```python
from build123d import *

# Parameters (mm, degrees)
CROQUIS1_R              = 3
SALIENTE_EXTRUIR1_DEPTH = 30
CROQUIS2_W              = 3.201408756
CROQUIS2_H              = 4
SALIENTE_EXTRUIR2_DEPTH = 9
REDONDEO2_R             = 1.5


with BuildPart() as part:
    # Croquis1 → Saliente-Extruir1 (new body)
    with BuildSketch(Plane(origin=(0, 0, 0), x_dir=(1, 0, 0), z_dir=(0, 1, 0))):
        with Locations(Location((0, 0, 0), (0, 0, 270))):
            Circle(CROQUIS1_R)
    extrude(amount=SALIENTE_EXTRUIR1_DEPTH)

    # Croquis2 → Saliente-Extruir2 (add)
    with BuildSketch(Plane.XY):
        with Locations((0, 28)):
            Rectangle(CROQUIS2_W, CROQUIS2_H)
    extrude(amount=SALIENTE_EXTRUIR2_DEPTH)

    # Redondeo2
    redondeo2_edges = [part.edges().sort_by_distance(p)[0] for p in [
        (1.600704378, 28, 9),
        (-1.600704378, 28, 9),
    ]]
    fillet(redondeo2_edges, radius=REDONDEO2_R)


solid = part.part
```
Geometry check sheet. Reference: the model listing, model coordinates, mm. A direction names the side the tool comes from. Give positions to 0.01 mm unless a question says otherwise; leave off trailing zeros. Order: outer loops, then holes, each group sorted by start corner. A loop starts at its lowest first (then second) coordinate and runs counter-clockwise, first axis right, second up.
1. Section check D-D, the plane z = 8. Enter the section's corners in (x, y), and give its area (3 significant figures).
2. Access from +Z, -Z, +X, -X, +Y, -Y to the whole of each face (thin tool, end or side, straight path). Record for faces 1 (the face through (0, 15, -3)), 2 (the face through (1.601, 28, 5)), 3 (the face through (-1.601, 28, 5)), 4 (the face through (0, 0, 0)), 5 (the face through (0, 30, 3)).
3. Thickness scan on L1, parallel to Z at x = -0.05, y = 19.5; L2, parallel to Y at x = 1, z = 3.5; L3, parallel to Z at x = 1, y = 23. Record the ranges inside material, lowest first.
4. Gauge pin test, flat ends, axial feed: pin 1 Ø2 at (x, y) = (0.5, 3.5) entering from -Z; pin 2 Ø3 at (y, z) = (27.5, 6) entering from +X; pin 3 Ø1.5 at (x, y) = (-2, 18) entering from -Z; pin 4 Ø2 at (y, z) = (27.5, 6) entering from -X. Record the tip position at first contact, or that the pin passes through.
5. Section check B-B, the plane y = 19.5. Enter the section's corners in (x, z).
6. Section check C-C, the plane z = 3.75. Enter the section's corners in (x, y), and give its area (3 significant figures).
7. Section check A-A, the plane x = -0.6. Enter the section's corners in (y, z), and give its area (3 significant figures).
Values follow:
1. outline: (-1.51, 26) - (1.51, 26) - (1.51, 30) - (-1.51, 30) - close
1. area: 12.1 mm2
2. face 1: -Y
2. face 2: +Z, +X, +Y, -Y
2. face 3: +Z, -X, +Y, -Y
2. face 4: +Z, -Z, +X, -X, -Y
2. face 5: +Z, -Z, +X, -X, +Y
3. L1: z = -3 to 3
3. L2: y = 26 to 30
3. L3: z = -2.83 to 2.83
4. pin 1: stops at z = -3
4. pin 2: stops at x = 1.6
4. pin 3: stops at z = -2.73
4. pin 4: stops at x = -1.6
5. outline: circle Ø6 at (0, 0)
6. outline: (-1.6, 26) - (1.6, 26) - (1.6, 30) - (-1.6, 30) - close
6. area: 12.8 mm2
7. outline: (0, -2.94) - (30, -2.94) - (30, 8.91) - (26, 8.91) - (26, 2.94) - (0, 2.94) - close
7. area: 200 mm2
